Read the model definition and answer for the solid it produces. Units are mm, in the model's axes. Coordinates: 2 decimals unless noted, no trailing zeros. Order: outer loops, then holes, each group sorted by start corner. A loop starts at its lowest first (then second) coordinate and runs counter-clockwise, first axis right, second up. Notation, with made-up numbers: M 56,-36 L 77,-36 A15 cw 77,-20 Z; hole C -23,58.5 d10. An arc over 180 degrees is marked long. Use a Markdown table: item, result. Add a question column.
1) The mould has two halves that part along X. Classify faces 1 (the face through (3.075, 1.479, -31.786)), 2 (the face through (18, 0, -18)), 3 (the face through (38, 1, -18)): released by +X, released by -X, zero draft, split by the parting line, or undercut.
2) Find the intervals of material crossed by probe 1 along Z at (x, y) = (2, 0.85); probe 2 along Z at (x, y) = (10, 1.8); probe 3 along X at (y, z) = (2.85, -34), in increasing order. Write a range as [from, to].
3) Find section B-B on z = -2.75. Write down the section's boundary in (x, y).
4) Find section A-A on x = 2.75. Write down the section's boundary in (y, z).
5) Find section C-C on y = 1.75. Count the separate pieces of the cut face and the enclosed holes in it, plus the area to 3 significant figures.
Autodesk Inventor part; units mm, degrees
ref_plane "YZ Plane" through (0, 0, 0) normal (1, 0, 0) x (0, 1, 0)
ref_plane "XZ Plane" through (0, 0, 0) normal (0, 1, 0) x (-1, 0, 0)
ref_plane "XY Plane" through (0, 0, 0) normal (0, 0, 1) x (1, 0, 0)
sketch "Sketch1" plane through (0, 0, 0) normal (0, 1, 0) x (-1, 0, 0)
  line L0 (0, 0) -> (-36, 0)
  line L1 (-36, 0) -> (-36, -36)
  line L2 (-36, -36) -> (0, -36)
  line L3 (0, -36) -> (0, 0)
  circle A0 centre (-10.5282, -25.3471) radius 1.5
  circle A1 centre (-25.4718, -25.3471) radius 1.5
  circle A2 centre (-10.5282, -10.6529) radius 1.5
  circle A3 centre (-25.4718, -10.6529) radius 1.5
  line L4 (2, -38) -> (2, 2)
  line L5 (2, 2) -> (-38, 2)
  line L6 (-38, 2) -> (-38, -38)
  line L7 (-38, -38) -> (2, -38)
  circle A4 centre (-2.75, -2.75) radius 1.5
  circle A5 centre (-33.25, -2.75) radius 1.5
  circle A6 centre (-33.25, -33.25) radius 1.5
  circle A7 centre (-2.75, -33.25) radius 1.5
  dimension "d0" = 36
  dimension "d1" = 36
  dimension "d50" = 40
  dimension "d51" = 40
  dimension "d55" = 3
  dimension "d56" = 3
  dimension "d57" = 3
  dimension "d58" = 3
extrude "Extrusion3" add sketch "Sketch1" along normal blind 3 contours L3 L2 L1 L0 | L7 L6 L5 L4
fillet "Fillet2" radius 2 4 edges at (38, 1.5, 2) (-2, 1.5, 2) (-2, 1.5, -38) (38, 1.5, -38)
properties part number "Topp"
Check result:
| question | item | result |
|---|---|---|
| 1 | face 1 | undercut |
| 1 | face 2 | zero draft |
| 1 | face 3 | released by +X |
| 2 | probe 1 | z = [-38, -34.55], [-31.95, -4.05], [-1.45, 2] |
| 2 | probe 2 | z = [-38, -26.75], [-23.94, -12.06], [-9.25, 2] |
| 2 | probe 3 | x = [-2, 1.45], [4.05, 31.95], [34.55, 38] |
| 3 | outline | M -2,0 L 1.25,0 L 1.25,3 L -2,3 Z; M 4.25,0 L 31.75,0 L 31.75,3 L 4.25,3 Z; M 34.75,0 L 38,0 L 38,3 L 34.75,3 Z |
| 4 | outline | M 0,-38 L 3,-38 L 3,-34.75 L 0,-34.75 Z; M 0,-31.75 L 3,-31.75 L 3,-4.25 L 0,-4.25 Z; M 0,-1.25 L 3,-1.25 L 3,2 L 0,2 Z |
| 5 | separate pieces | 1 |
| 5 | enclosed holes | 8 |
| 5 | area | 1,540 mm2 |
